The model under review builds one solid part; all positions refer to its coordinate system, in mm. Round coordinates to 2 decimals unless told otherwise and drop trailing zeros. Write each loop counter-clockwise with the first axis right and the second up, starting at its lowest first coordinate (ties: lowest second). Pieces come first, ordered by that corner, then holes. Notation, with made-up numbers: (-13.75, -22.75) -> (39.25, -22.75) arc R33 ccw to (39.25, 11.25) -> close; hole circle Ø10 at (63, 49). An arc over 180 degrees is marked (long way). Answer as a JSON object with one key per item and string values. Group by question number.
1) To check wall thickness, follow probe 1 along Z at (x, y) = (0, 2.55); probe 2 along Z at (x, y) = (3.25, 2.9); probe 3 along X at (y, z) = (4.1, -2.5). State the ranges of each line that lie inside material, in increasing order. Write a range as [from, to].
2) We need section B-B, the plane z = 0. Write out the cut boundary in (x, y).
3) We need section C-C, the plane y = 2.2. Write out the cut boundary in (x, z), then the cut area to 3 significant figures.
4) Mouldability with a two-part tool opening along X and no side actions: class faces 1 (the cylindrical face through (-0.867, 2.465, -3.905)), 2 (the flat face through (0, 2, -10)), 3 (the flat face through (5, 2, 0)) as pulls with the +X half, pulls with the -X half, needs draft (parallel to the pull), parting line crosses it, or undercut.
5) We need section A-A, the plane x = 0. Write out the cut boundary in (y, z), then the cut area to 3 significant figures.
Solid Edge part; units mm, degrees
sketch "Sketch1" plane through (0, 0, 0) normal (0, -1, 0) x (1, 0, 0)
  circle A0 centre (0, 0) radius 4
  line L0 (5, 10) -> (-5, 10)
  line L1 (-5, 10) -> (-5, -10)
  line L2 (-5, -10) -> (5, -10)
  line L3 (5, -10) -> (5, 10)
extrude "Protrusion1" add sketch "Sketch1" against normal blind 5
Here are the results:
{
 "1": {"probe 1": "z = [-10, -4], [4, 10]", "probe 2": "z = [-10, -2.33], [2.33, 10]", "probe 3": "x = [-5, -3.12], [3.12, 5]"},
 "2": {"outline": "(-5, 0) -> (-4, 0) -> (-4, 5) -> (-5, 5) -> close; (4, 0) -> (5, 0) -> (5, 5) -> (4, 5) -> close"},
 "3": {"outline": "(-5, -10) -> (5, -10) -> (5, 10) -> (-5, 10) -> close; hole circle Ø8 at (0, 0)", "area": "150 mm^2"},
 "4": {"face 1": "undercut", "face 2": "needs draft", "face 3": "pulls with the +X half"},
 "5": {"outline": "(0, -10) -> (5, -10) -> (5, -4) -> (0, -4) -> close; (0, 4) -> (5, 4) -> (5, 10) -> (0, 10) -> close", "area": "60.0 mm^2"}
}
